```python
from build123d import *

# Parameters (mm, degrees)
BOSS_EXTRUDE1_DEPTH  = 10
FILLET1_R            = 5
M3_CLEARANCE_HOLE1_D = 3.6
M3_CLEARANCE_HOLE2_D = 3.6


with BuildPart() as part:
    # Sketch3 → Boss-Extrude1 (new body)
    with BuildSketch(Plane.XY):
        with BuildLine():
            Line((0, 0), (-30, 0))
            ThreePointArc((-30, 0), (-44.142135624, 5.857864376), (-50, 20))
            Line((-50, 20), (-50, 71.627417))
            Line((-50, 71.627417), (-45, 71.627417))
            Line((-45, 71.627417), (-45, 20))
            ThreePointArc((-45, 20), (-40.606601718, 9.393398282), (-30, 5))
            Line((-30, 5), (0, 5))
            Line((0, 5), (0, 0))
        make_face()
    extrude(amount=BOSS_EXTRUDE1_DEPTH)

    # Fillet1
    fillet1_edges = [part.edges().sort_by_distance(p)[0] for p in [
        (0, 2.5, 10),
        (0, 2.5, 0),
        (-47.5, 71.627417, 0),
        (-47.5, 71.627417, 10),
    ]]
    fillet(fillet1_edges, radius=FILLET1_R - 0.0001)  # a hair under: the kernel refuses the full size

    # M3 Clearance Hole1 (through all)
    with Locations(Plane.XZ):
        with Locations((-5, 5)):
            Hole(M3_CLEARANCE_HOLE1_D / 2)

    # M3 Clearance Hole2 (through all)
    with Locations(Plane.ZY.offset(50)):
        with Locations((5, 66.627417)):
            Hole(M3_CLEARANCE_HOLE2_D / 2)


solid = part.part
```
Source: CAD feature listing. Evaluate the final solid. Frame: model axes, mm. A direction names the side the tool comes from. Coordinates: 2 decimals unless noted, no trailing zeros. Loops run counter-clockwise (first coordinate to the right, second up) from the corner with the lowest first, then second, coordinate; pieces in that order, holes last. Notation, with made-up numbers: M 35,12.5 L 50,12.5 A18 cw 50,29.5 Z; hole C 85,-32 d3. An arc over 180 degrees is marked long. Put each result on its own line as item: value. Start each with the question number.
1) Pull-direction query (Y, two-part tool) for faces 1 (the face through (-47.465, 68.412, 5.234)), 2 (the face through (-47.5, 70.2, 1.5)), 3 (the face through (-45, 46, 5)); classes: pulls with the +Y half, pulls with the -Y half, needs draft (parallel to the pull), parting line crosses it, or undercut.
2) Ray query, L1, parallel to Z at x = -5, y = 2.9; L2, parallel to Y at x = -25, z = 8; L3, parallel to X at y = 33, z = 6.5. Return the intervals inside material, ascending. Write a range as from..to.
3) Cut plane C-C on y = 51. Return the cut outline in (x, z).
4) Cut plane B-B on x = -13. Return the cut outline in (y, z).
5) Cut plane A-A on z = 4.25. Return the cut outline in (x, y), then the cut area to 3 significant figures.
6) Contact query for flat-ended pins moving along their axis: pin 1 Ø3 at (y, z) = (23.5, 5.5) entering from +X; pin 2 Ø3 at (x, z) = (-20, 3) entering from +Y. Output: stop coordinate, or through.
7) Reachability of faces 4 (the face through (-46, 24, 0)), 5 (the face through (-15, 5, 5)) from +Z, -Z, +X, -X, +Y, -Y: full face, straight path, thin tool, end or side. Return the list, or none.
The answers:
1. face 1: undercut
1. face 2: pulls with the +Y half
1. face 3: needs draft
2. L1: z = 0..3.2, 6.8..10
2. L2: y = 0..5
2. L3: x = -50..-45
3. outline: M -50,0 L -45,0 L -45,10 L -50,10 Z
4. outline: M 0,0 L 5,0 L 5,10 L 0,10 Z
5. outline: M -50,20 A20 ccw -30,0 L -6.64,0 L -6.64,5 L -30,5 A15 cw -45,20 L -45,64.99 L -50,64.99 Z; M -50,68.26 L -45,68.26 L -45,71.57 L -50,71.57 Z; M -3.36,0 L -0.06,0 L -0.06,5 L -3.36,5 Z
5. area: 512 mm²
6. pin 1: stops at x = -45
6. pin 2: stops at y = 5
7. face 4: -Z, +X, -X, +Y, -Y
7. face 5: +Z, -Z, +X, +Y
